Part print with two shaded views. Sizes in mm from the minimum x, y, z corner. A direction names the side the tool comes from. Round coordinates to 2 decimals unless told otherwise and drop trailing zeros. Order: outer loops, then holes, each group sorted by start corner. A loop starts at its lowest first (then second) coordinate and runs counter-clockwise, first axis right, second up. Notation, with made-up numbers: M 14.25,-9.5 L 30.25,-9.5 A21 cw 30.25,22.5 Z; hole C 65.5,37.25 d9. An arc over 180 degrees is marked long. Put each result on its own line as item: value.
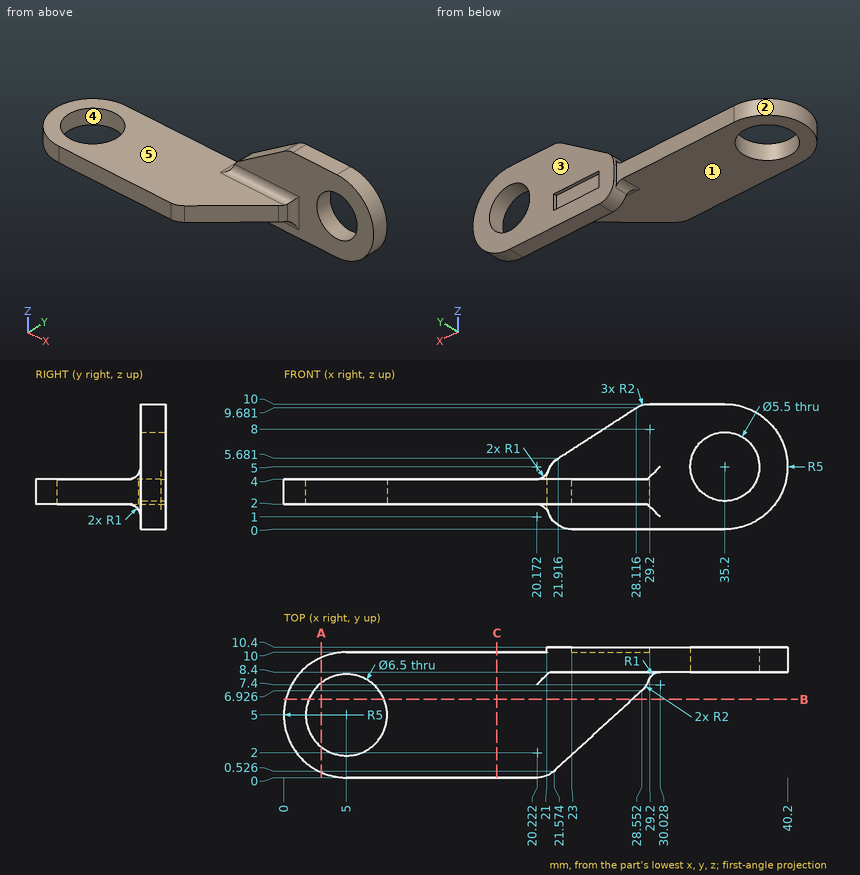
Item 1: Mould opens along Y. For the marked faces 3, 4 and 5 say: pulls with the +Y half, pulls with the -Y half, needs draft (parallel to the pull), parting line crosses it, or undercut.
Answers below:
face 3: pulls with the +Y half
face 4: undercut
face 5: needs draft
Item 2: Tool access for the marked faces 1 and 2: list every direction of +Z, -Z, +X, -X, +Y, -Y with a clear straight run to the whole face (end or side of a thin tool).
Answers below:
face 1: -Z, -X, -Y
face 2: +Z, -Z, -X
Item 3: Band-saw the part on C-C on x = 17. Give the cut face in (y, z), and give its area (3 significant figures).
Answers below:
outline: M 0,2 L 10,2 L 10,4 L 0,4 Z
area: 20.0 mm²
Item 4: Probe line 1 along X through (y, z) = (9.15, 5); line 2 along Z through (x, y) = (8, 9); line 3 along X through (y, z) = (4, 3.25) (1 decimal). List the from-to ranges inside material, lowest first. Write a range as [from, to].
Answers below:
line 1: [21.27, 32.45], [37.95, 40.2]
line 2: [2, 4]
line 3: [0.1, 1.9], [8.1, 25.4]
Item 5: Band-saw the part on B-B on y = 6.25. Give the cut face in (x, z) (1 decimal).
Answers below:
outline: M 0.2,2 L 2,2 L 2,4 L 0.2,4 Z; M 8,2 L 27.8,2 L 27.8,4 L 8,4 Z
Item 6: Pin check, flat tips, straight feed: P1, Ø5, axis at x = 6.5, y = 7, coming from the +Z side; P2, Ø1, axis at x = 10, z = 4, coming from the +Y side; P3, Ø6, axis at x = 33.5, z = 1.5, coming from the -Y side; P4, Ø5, axis at y = 4.5, z = 3.5, coming from the -X side. Stop position of each tip, or through.
Answers below:
P1: z = 4
P2: y = 10
P3: y = 8.4
P4: x = 0
Item 7: Band-saw the part on A-A on x = 3. Give the cut face in (y, z).
Answers below:
outline: M 0.42,2 L 2.44,2 L 2.44,4 L 0.42,4 Z; M 7.56,2 L 9.58,2 L 9.58,4 L 7.56,4 Z
